Part model, mm, in its own coordinate system. Face numbers are marked on the shaded views. Round coordinates to 2 decimals unless told otherwise and drop trailing zeros. Loops run counter-clockwise (first coordinate to the right, second up) from the corner with the lowest first, then second, coordinate; pieces in that order, holes last. Notation, with made-up numbers: M 36.5,16.5 L 76.5,16.5 A21 cw 76.5,43.5 Z; hole C -4,87 d5. An arc over 180 degrees is marked long. Answer as CSV lines item,"result". Start each with the question number.
Item 1: Band-saw the part on B-B (z = 20). Give the cut face in (x, y), and give its area (3 significant figures).
Item 2: Band-saw the part on A-A (z = 3.75). Give the cut face in (x, y).
Item 3: Mould opens along X. For the marked faces 1, 2, 3 and 4 say: pulls with the +X half, pulls with the -X half, needs draft (parallel to the pull), parting line crosses it, or undercut.
Item 4: Wall check: line 1 (X direction, y = -3, z = 16); line 2 (Y direction, x = 26, z = 7.5); line 3 (X direction, y = -21, z = 14). Give the ranges that are in metal, low to high.
```python
from build123d import *

# Parameters (mm, degrees)
F0_W     = 86.9801938534
F0_H     = 75.3522887826
F0_R     = 32.2813153837
F1_DEPTH = 25.4
F3_R     = 5.08


# Not quite as in the source:
# - a fillet or chamfer that OpenCascade refuses, or shapes differently, is made with other operations: its cross-section is extruded or revolved along the edge and cut away or added


with BuildPart() as f1:
    # F0 (on Top) → F1 (new body)
    with BuildSketch(Plane.XY):
        with Locations((13.0896866322, -5.9322379529)):
            Rectangle(F0_W, F0_H)
        with Locations((13.0896866322, -5.9322379529)):
            Circle(F0_R, mode=Mode.SUBTRACT)
    extrude(amount=F1_DEPTH)

    # F2: fillet of radius 6.35 on 1 edges, made by hand

    # F2_s1 → F2_t2 (revolve, cut)
    with BuildSketch(Plane.XZ.offset(5.9322379529)):
        with BuildLine():
            ThreePointArc((45.3710020159, 19.05), (47.2308739553, 23.5401280605), (51.7210020159, 25.4))
            Line((51.7210020159, 25.4), (45.3710020159, 25.4))
            Line((45.3710020159, 25.4), (45.3710020159, 19.05))
        make_face()
    revolve(axis=Axis((13.0896866322, -5.9322379529, 25.4), (0, 0, 1)), mode=Mode.SUBTRACT)

    # F3
    f3_edges = [f1.edges().sort_by_distance(p)[0] for p in [
        (-19.191629, -5.932238, 0),
    ]]
    fillet(f3_edges, radius=F3_R)


solid = f1.part
```
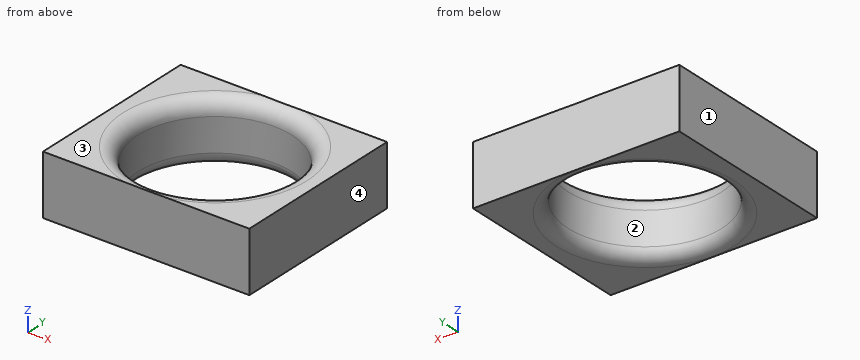
Answer block:
1,outline,"M -30.4,-43.61 L 56.58,-43.61 L 56.58,31.74 L -30.4,31.74 Z; hole C 13.09,-5.93 d64.71"
1,area,"3,270 mm^2"
2,outline,"M -30.4,-43.61 L 56.58,-43.61 L 56.58,31.74 L -30.4,31.74 Z; hole C 13.09,-5.93 d64.92"
3,face 1,"pulls with the -X half"
3,face 2,"undercut"
3,face 3,"needs draft"
3,face 4,"pulls with the +X half"
4,line 1,"x = -30.4 to -19.06, 45.24 to 56.58"
4,line 2,"y = -43.61 to -35.52, 23.66 to 31.74"
4,line 3,"x = -30.4 to -15.46, 41.64 to 56.58"
